from build123d import *

# Parameters (mm, degrees)
F1_DEPTH = 12.7
F3_D     = 7.5946
F5_DEPTH = 25.4


with BuildPart() as f1:
    # F0 (on Front) → F1 (new body)
    with BuildSketch(Plane.XZ):
        Polygon((-23.688762, 0), (-1.933777, 0), (1.772629, 0), (11.602659, -7.976828), (19.337766, -27.798036), (23.608761, -21.086473), (24.058953, -17.065071), (19.337766, -5.253581), (9.385022, 4.699161), (4.234401, 7.976828), (-21.754986, 7.976828), (-37.24273, 0), (-37.547495, -7.976828), align=None)
    extrude(amount=F1_DEPTH)

    # F3 (through all)
    with Locations(Plane.XZ.offset(12.7)):
        with Locations((18.250674, -14.809974)):
            Hole(F3_D / 2)

    # F4 (on face) → F5 (cut)
    with BuildSketch(Plane.XZ.offset(12.7)):
        with BuildLine():
            ThreePointArc((23.785793, -16.381676), (20.622019, -19.575228), (16.126665, -19.569593))
            Line((16.126665, -19.569593), (19.337766, -27.798036))
            Line((19.337766, -27.798036), (23.608761, -21.086473))
            Line((23.608761, -21.086473), (24.058953, -17.065071))
            Line((24.058953, -17.065071), (23.785793, -16.381676))
        make_face()
    extrude(amount=-F5_DEPTH, mode=Mode.SUBTRACT)


solid = f1.part
Input: part model. Units: mm. Frame: model coordinates. A direction names the side the tool comes from. Give positions to 0.01 mm unless a question says otherwise; leave off trailing zeros. Order: outer loops, then holes, each group sorted by start corner. A loop starts at its lowest first (then second) coordinate and runs counter-clockwise, first axis right, second up. Notation, with made-up numbers: (81.5, 58.5) - (95.5, 58.5) arc R26 ccw to (95.5, 75.5) - close; hole circle Ø5 at (13, 18). An arc over 180 degrees is marked (long way). Answer as a JSON object with one key per item and string values. Group by question number.
Q1. First-contact query: pin 1 Ø4.5 at (x, z) = (18.25, -14.81) entering from -Y; pin 2 Ø2 at (y, z) = (-8, -2.5) entering from +X; pin 3 Ø5 at (y, z) = (-11, -9) entering from +X; pin 4 Ø1 at (y, z) = (-8.5, -14) entering from +X. Flat tips, straight axial feed; report the tip coordinate or a pass-through.
Q2. Line query: probe 1 along Z at (x, y) = (-21, -12); probe 2 along X at (y, z) = (-2.5, -0.5); probe 3 along X at (y, z) = (-4, -1.75). Output: solid intervals per line, ascending.
Q3. Cut plane C-C, the plane x = -4.5. Output: boundary loops of the cut face in (y, z).
Q4. Mould query, pull axis X, two halves, no side actions, for faces 1 (the face through (15.6, -6.26, -18.22)), 2 (the face through (21.593, -6.261, -10.896)), 3 (the face through (21.73, -6.26, -13.29)). Classes: pulls with the +X half, pulls with the -X half, needs draft (parallel to the pull), parting line crosses it, or undercut.
Q5. Cut plane A-A, the plane z = -12.5. Output: boundary loops of the cut face in (x, y), then the cut area to 3 significant figures.
Q6. Cut plane D-D, the plane z = -17.75. Output: boundary loops of the cut face in (x, y), then the cut area to 3 significant figures.
Q7. Cut plane B-B, the plane y = -10.5. Output: boundary loops of the cut face in (x, z), then the cut area to 3 significant figures.
Q8. Set-up query: faces 4 (the face through (-9, -6, 7.977)), 5 (the face through (-11, -6, 0)). Return all of +Z, -Z, +X, -X, +Y, -Y with unobstructed straight access to the full face (end or side cutting, diameter ignored); none if empty.
Results:
{
 "1": {"pin 1": "through", "pin 2": "x = 17.58", "pin 3": "x = 21.83", "pin 4": "x = 23.03"},
 "2": {"probe 1": "0 to 7.98", "probe 2": "-37.26 to -24.56, 2.39 to 14.58", "probe 3": "-37.31 to -26.73, 3.93 to 15.83"},
 "3": {"outline": "(-12.7, 0) - (0, 0) - (0, 7.98) - (-12.7, 7.98) - close"},
 "4": {"face 1": "pulls with the -X half", "face 2": "pulls with the +X half", "face 3": "undercut"},
 "5": {"outline": "(13.37, -12.7) - (15.24, -12.7) - (15.24, 0) - (13.37, 0) - close; (21.26, -12.7) - (22.23, -12.7) - (22.23, 0) - (21.26, 0) - close", "area": "36.1 mm^2"},
 "6": {"outline": "(15.42, -12.7) - (15.85, -12.7) - (15.85, 0) - (15.42, 0) - close; (20.65, -12.7) - (23, -12.7) - (23, 0) - (20.65, 0) - close", "area": "35.3 mm^2"},
 "7": {"outline": "(-37.55, -7.98) - (-23.69, 0) - (1.77, 0) - (11.6, -7.98) - (14.5, -15.4) arc R3.8 cw (long way) to (15.09, -16.92) - (16.13, -19.57) arc R5.83 ccw to (23.79, -16.38) - (19.34, -5.25) - (9.39, 4.7) - (4.23, 7.98) - (-21.75, 7.98) - (-37.24, 0) - close", "area": "509 mm^2"},
 "8": {"face 4": "+Z, +X, -X, +Y, -Y", "face 5": "-Z, +Y, -Y"}
}
